Check sheet for the drawn part. Datum: minimum x, y, z corner. Units: mm. A direction names the side the tool comes from. Round coordinates to 2 decimals unless told otherwise and drop trailing zeros. Write each loop counter-clockwise with the first axis right and the second up, starting at its lowest first coordinate (ties: lowest second). Pieces come first, ordered by that corner, then holes.
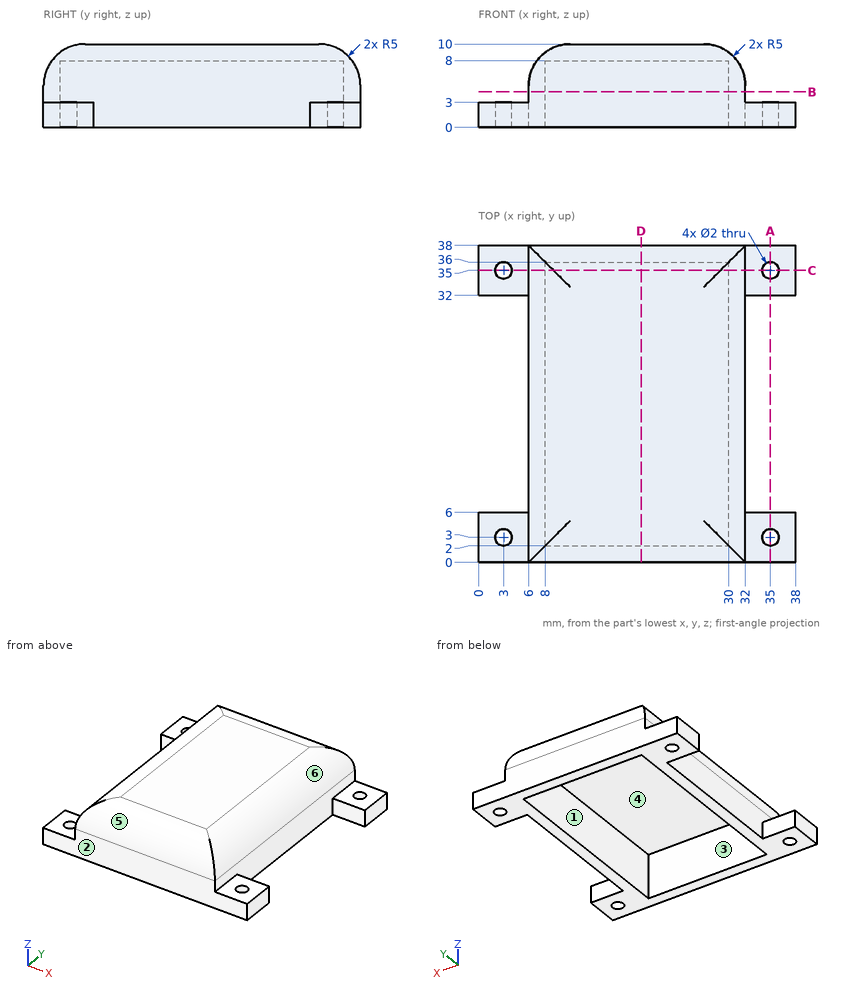
Q1. Sectioned sample at A-A (x = 35). Enter the section's corners in (y, z), plus the area to 3 significant figures.
Recorded:
outline: (0, 0) - (2, 0) - (2, 3) - (0, 3) - close; (4, 0) - (6, 0) - (6, 3) - (4, 3) - close; (32, 0) - (34, 0) - (34, 3) - (32, 3) - close; (36, 0) - (38, 0) - (38, 3) - (36, 3) - close
area: 24.0 mm2
Q2. Tool access check on the marked faces 1 and 2. Record the directions out of +Z, -Z, +X, -X, +Y, -Y that give a thin tool (end or side, any length) a straight path to the whole face; none if there is none.
Recorded:
face 1: -Z
face 2: +Z, -Z, +X, -X, -Y
Q3. Sectioned sample at B-B (z = 4.25). Enter the section's corners in (x, y), plus the area to 3 significant figures.
Recorded:
outline: (6, 0) - (32, 0) - (32, 38) - (6, 38) - close; hole (8, 2) - (30, 2) - (30, 36) - (8, 36) - close
area: 240 mm2
Q4. Depth check by flat-ended pin: P1, Ø11, axis at x = 23.5, y = 16.5, coming from the -Z side; P2, Ø4, axis at x = 6, z = 9, coming from the +Y side; P3, Ø5.5, axis at y = 23.5, z = 1.5, coming from the +X side. Enter the tip coordinate at first touch or a pass-through.
Recorded:
P1: stops at z = 8
P2: stops at y = 37.56
P3: stops at x = 32
Q5. Release check for a two-part mould opening along Y. For the marked faces 3, 4, 5 and 6 record: released by +Y, released by -Y, zero draft, split by the parting line, or undercut.
Recorded:
face 3: undercut
face 4: undercut
face 5: released by -Y
face 6: zero draft
Q6. Sectioned sample at C-C (y = 35). Enter the section's corners in (x, z), plus the area to 3 significant figures.
Recorded:
outline: (0, 0) - (2, 0) - (2, 3) - (0, 3) - close; (4, 0) - (8, 0) - (8, 8) - (30, 8) - (30, 0) - (34, 0) - (34, 3) - (32, 3) - (32, 5) arc R5 ccw to (29, 9.58) - (9, 9.58) arc R5 ccw to (6, 5) - (6, 3) - (4, 3) - close; (36, 0) - (38, 0) - (38, 3) - (36, 3) - close
area: 89.5 mm2
Q7. Material ranges on line 1 along X through (y, z) = (35, 1.5); line 2 along Y through (x, z) = (35, 1.3); line 3 along X through (y, z) = (18, 4), recorded low to high.
Recorded:
line 1: x = 0 to 2, 4 to 8, 30 to 34, 36 to 38
line 2: y = 0 to 2, 4 to 6, 32 to 34, 36 to 38
line 3: x = 6 to 8, 30 to 32
Q8. Sectioned sample at D-D (x = 19.5). Enter the section's corners in (y, z), plus the area to 3 significant figures.
Recorded:
outline: (0, 0) - (2, 0) - (2, 8) - (36, 8) - (36, 0) - (38, 0) - (38, 5) arc R5 ccw to (33, 10) - (5, 10) arc R5 ccw to (0, 5) - close
area: 97.3 mm2
